For this review, take the finished solid that the model builds, in its own axes (mm). A direction names the side the tool comes from. Coordinates: 2 decimals unless noted, no trailing zeros. Order: outer loops, then holes, each group sorted by start corner. A loop starts at its lowest first (then second) coordinate and runs counter-clockwise, first axis right, second up. Notation, with made-up numbers: M 46.5,56.25 L 95.5,56.25 A22 ccw 95.5,63.25 Z; hole C 2,31.5 d4. An arc over 180 degrees is marked long. Use CSV: the item, a comma, the result in double quotes.
```python
from build123d import *

# Parameters (mm, degrees)
SKETCH1_W           = 109
SKETCH1_H           = 14
BOSS_EXTRUDE1_DEPTH = 3
SKETCH2_W           = 88.121085129
SKETCH2_H           = 14
BOSS_EXTRUDE2_DEPTH = 3
SKETCH3_R           = 1.6
CUT_EXTRUDE1_DEPTH  = 3
SKETCH4_W           = 19.094363251
SKETCH4_H           = 13.060900744
SKETCH4_W_2         = 19.108315111
CUT_EXTRUDE2_DEPTH  = 6
SKETCH5_W           = 10.384994466
SKETCH5_H           = 3
SKETCH5_W_2         = 10.493920405
BOSS_EXTRUDE3_DEPTH = 2


with BuildPart() as part:
    # Sketch1 → Boss-Extrude1 (new body)
    with BuildSketch(Plane(origin=(0, 0, 0), x_dir=(1, 0, 0), z_dir=(0, 1, 0))):
        with Locations((54.5, 7)):
            Rectangle(SKETCH1_W, SKETCH1_H)
    extrude(amount=BOSS_EXTRUDE1_DEPTH)

    # Sketch2 → Boss-Extrude2 (add)
    with BuildSketch(Plane(origin=(0, 3, 0), x_dir=(1, 0, 0), z_dir=(0, 1, 0))):
        with Locations((54.44553703, 7)):
            Rectangle(SKETCH2_W, SKETCH2_H)
    extrude(amount=BOSS_EXTRUDE2_DEPTH)

    # Sketch3 → Cut-Extrude1 (cut)
    with BuildSketch(Plane(origin=(0, 3, 0), x_dir=(1, 0, 0), z_dir=(0, 1, 0))):
        with Locations(Location((5.192497233, 7, 0), (0, 0, 270))):
            Circle(SKETCH3_R)
        with Locations(Location((103.753039797, 7, 0), (0, 0, 270))):
            Circle(SKETCH3_R)
    extrude(amount=-CUT_EXTRUDE1_DEPTH, mode=Mode.SUBTRACT)

    # Sketch4 → Cut-Extrude2 (cut)
    with BuildSketch(Plane(origin=(0, 6, 0), x_dir=(1, 0, 0), z_dir=(0, 1, 0))):
        with Locations((83.937166007, 6.530450372)):
            Rectangle(SKETCH4_W, SKETCH4_H)
        with Locations((24.977978122, 6.530450372)):
            Rectangle(SKETCH4_W_2, SKETCH4_H)
    extrude(amount=-CUT_EXTRUDE2_DEPTH, mode=Mode.SUBTRACT)

    # Sketch5 → Boss-Extrude3 (add)
    with BuildSketch(Plane(origin=(0, 0, -14), x_dir=(-1, 0, 0), z_dir=(0, 0, -1))):
        Polygon((-98.506079595, 0), (-10.384994466, 0), (-10.384994466, 3), (-10.384994466, 6), (-98.506079595, 6), (-98.506079595, 3), align=None)
        with Locations((-5.192497233, 1.5)):
            Rectangle(SKETCH5_W, SKETCH5_H)
        with Locations((-103.753039798, 1.5)):
            Rectangle(SKETCH5_W_2, SKETCH5_H)
    extrude(amount=BOSS_EXTRUDE3_DEPTH)


solid = part.part
```
Item 1: Draft analysis for pull direction X (two halves, no side actions). For faces 4 (the face through (104, 3, -10)), 5 (the face through (15.424, 3, -6)), 6 (the face through (109, 1, -8)), 7 (the face through (10.385, 4, -8)), state which applies: released by +X, released by -X, zero draft, split by the parting line, or undercut.
Solutions:
face 4,"zero draft"
face 5,"undercut"
face 6,"released by +X"
face 7,"released by -X"
Item 2: Add section A-A on z = -11.5. State the section outline as (x, y) points (3 decimals), and give its area (3 significant figures).
Solutions:
outline,"M 0,0 L 15.424,0 L 15.424,6 L 10.385,6 L 10.385,3 L 0,3 Z; M 34.532,0 L 74.39,0 L 74.39,6 L 34.532,6 Z; M 93.484,0 L 109,0 L 109,3 L 98.506,3 L 98.506,6 L 93.484,6 Z"
area,"362 mm^2"
Item 3: Clearance check with flat-ended pins moving along their axes: pin 1 Ø2.5 at (x, z) = (5.19, -7) entering from +Y; pin 2 Ø5 at (x, z) = (3, -8.5) entering from +Y; pin 3 Ø2 at (y, z) = (4.5, -5.5) entering from -X (3 decimals); pin 4 Ø1.5 at (y, z) = (4, -8.5) entering from +X. State where each tip first meets the part, or that it passes through.
Solutions:
pin 1,"through"
pin 2,"y = 3"
pin 3,"x = 10.385"
pin 4,"x = 98.51"
Item 4: For faces 1 (the face through (84, 3, -13.061)), 2 (the face through (98.506, 5, -8)), 3 (the face through (5, 3, -10)), list the 3-axis set-ups (+Z, -Z, +X, -X, +Y, -Y) from which the entire face can be reached by the end or side of a thin tool; tool diameter is ignored.
Solutions:
face 1,"+Z, +Y, -Y"
face 2,"+Z, -Z, +X, +Y"
face 3,"+Z, -Z, -X, +Y"
Item 5: To check wall thickness, follow line 1 along X through (y, z) = (4.6, -3.5) (3 decimals); line 2 along X through (y, z) = (2.2, -7); line 3 along X through (y, z) = (2.8, -13). State the ranges of each line that lie inside material, in increasing order. Write a range as [from, to].
Solutions:
line 1,"[10.385, 15.424], [34.532, 74.39], [93.484, 98.506]"
line 2,"[0, 3.59], [6.79, 15.42], [34.53, 74.39], [93.48, 102.15], [105.35, 109]"
line 3,"[0, 15.42], [34.53, 74.39], [93.48, 109]"
Item 6: Add section B-B on z = -7. State the section outline as (x, y) points (1 decimal), and give its area (3 significant figures).
Solutions:
outline,"M 0,0 L 3.6,0 L 3.6,3 L 0,3 Z; M 6.8,0 L 15.4,0 L 15.4,6 L 10.4,6 L 10.4,3 L 6.8,3 Z; M 34.5,0 L 74.4,0 L 74.4,6 L 34.5,6 Z; M 93.5,0 L 102.2,0 L 102.2,3 L 98.5,3 L 98.5,6 L 93.5,6 Z; M 105.4,0 L 109,0 L 109,3 L 105.4,3 Z"
area,"343 mm^2"
Item 7: Add section C-C on x = 99.5. State the section outline as (y, z) points, and give its area (3 significant figures).
Solutions:
outline,"M 0,-16 L 3,-16 L 3,0 L 0,0 Z"
area,"48.0 mm^2"
